```python
from build123d import *

# Parameters (mm, degrees)
BOSS_EXTRUDE1_DEPTH = 10
FILLET1_R           = 2


with BuildPart() as part:
    # Sketch1 → Boss-Extrude1 (new body)
    with BuildSketch(Plane.XY):
        with BuildLine():
            ThreePointArc((-10.758537028, -9.344323465), (-14.25, 0), (-10.758537028, 9.344323465))
            Line((-10.758537028, 9.344323465), (-15, 13.585786438))
            Line((-15, 13.585786438), (-15, -13.585786438))
            Line((-15, -13.585786438), (-10.758537028, -9.344323465))
        make_face()
        with BuildLine():
            ThreePointArc((-9.344323465, -10.758537028), (-10.076271632, -10.076271632), (-10.758537028, -9.344323465))
            Line((-10.758537028, -9.344323465), (-15, -13.585786438))
            Line((-15, -13.585786438), (-15, -15))
            Line((-15, -15), (-13.585786438, -15))
            Line((-13.585786438, -15), (-9.344323465, -10.758537028))
        make_face()
        with BuildLine():
            ThreePointArc((9.344323465, -10.758537028), (0, -14.25), (-9.344323465, -10.758537028))
            Line((-9.344323465, -10.758537028), (-13.585786438, -15))
            Line((-13.585786438, -15), (13.585786438, -15))
            Line((13.585786438, -15), (9.344323465, -10.758537028))
        make_face()
        with BuildLine():
            Line((15, -15), (15, -13.585786438))
            Line((15, -13.585786438), (10.758537028, -9.344323465))
            ThreePointArc((10.758537028, -9.344323465), (10.076271632, -10.076271632), (9.344323465, -10.758537028))
            Line((9.344323465, -10.758537028), (13.585786438, -15))
            Line((13.585786438, -15), (15, -15))
        make_face()
        with BuildLine():
            Line((15, 13.585786438), (10.758537028, 9.344323465))
            ThreePointArc((10.758537028, 9.344323465), (13.348626383, 4.987652121), (14.25, 0))
            ThreePointArc((14.25, 0), (13.348626383, -4.987652121), (10.758537028, -9.344323465))
            Line((10.758537028, -9.344323465), (15, -13.585786438))
            Line((15, -13.585786438), (15, 13.585786438))
        make_face()
        with BuildLine():
            Line((15, 15), (13.585786438, 15))
            Line((13.585786438, 15), (9.344323465, 10.758537028))
            ThreePointArc((9.344323465, 10.758537028), (10.076271632, 10.076271632), (10.758537028, 9.344323465))
            Line((10.758537028, 9.344323465), (15, 13.585786438))
            Line((15, 13.585786438), (15, 15))
        make_face()
        with BuildLine():
            Line((13.585786438, 15), (-13.585786438, 15))
            Line((-13.585786438, 15), (-9.344323465, 10.758537028))
            ThreePointArc((-9.344323465, 10.758537028), (0, 14.25), (9.344323465, 10.758537028))
            Line((9.344323465, 10.758537028), (13.585786438, 15))
        make_face()
        with BuildLine():
            Line((-9.344323465, 10.758537028), (-13.585786438, 15))
            Line((-13.585786438, 15), (-15, 15))
            Line((-15, 15), (-15, 13.585786438))
            Line((-15, 13.585786438), (-10.758537028, 9.344323465))
            ThreePointArc((-10.758537028, 9.344323465), (-10.076271632, 10.076271632), (-9.344323465, 10.758537028))
        make_face()
        with BuildLine():
            Line((3.83436875, -5.248582312), (0, -1.414213562))
            Line((0, -1.414213562), (-3.83436875, -5.248582312))
            ThreePointArc((-3.83436875, -5.248582312), (0, -6.5), (3.83436875, -5.248582312))
        make_face()
        with BuildLine():
            Line((0, -1.414213562), (-1.414213562, 0))
            Line((-1.414213562, 0), (-5.248582312, -3.83436875))
            ThreePointArc((-5.248582312, -3.83436875), (-4.596194078, -4.596194078), (-3.83436875, -5.248582312))
            Line((-3.83436875, -5.248582312), (0, -1.414213562))
        make_face()
        with BuildLine():
            Line((-1.414213562, 0), (-5.248582312, 3.83436875))
            ThreePointArc((-5.248582312, 3.83436875), (-6.5, 0), (-5.248582312, -3.83436875))
            Line((-5.248582312, -3.83436875), (-1.414213562, 0))
        make_face()
        with BuildLine():
            Line((0, 1.414213562), (-3.83436875, 5.248582312))
            ThreePointArc((-3.83436875, 5.248582312), (-4.596194078, 4.596194078), (-5.248582312, 3.83436875))
            Line((-5.248582312, 3.83436875), (-1.414213562, 0))
            Line((-1.414213562, 0), (0, 1.414213562))
        make_face()
        with BuildLine():
            ThreePointArc((3.83436875, 5.248582312), (0, 6.5), (-3.83436875, 5.248582312))
            Line((-3.83436875, 5.248582312), (0, 1.414213562))
            Line((0, 1.414213562), (3.83436875, 5.248582312))
        make_face()
        with BuildLine():
            Line((3.83436875, 5.248582312), (0, 1.414213562))
            Line((0, 1.414213562), (1.414213562, 0))
            Line((1.414213562, 0), (5.248582312, 3.83436875))
            ThreePointArc((5.248582312, 3.83436875), (4.596194078, 4.596194078), (3.83436875, 5.248582312))
        make_face()
        with BuildLine():
            Line((5.248582312, 3.83436875), (1.414213562, 0))
            Line((1.414213562, 0), (5.248582312, -3.83436875))
            ThreePointArc((5.248582312, -3.83436875), (6.179230738, -2.01670709), (6.5, 0))
            ThreePointArc((6.5, 0), (6.179230738, 2.01670709), (5.248582312, 3.83436875))
        make_face()
        with BuildLine():
            Line((5.248582312, -3.83436875), (1.414213562, 0))
            Line((1.414213562, 0), (0, -1.414213562))
            Line((0, -1.414213562), (3.83436875, -5.248582312))
            ThreePointArc((3.83436875, -5.248582312), (4.596194078, -4.596194078), (5.248582312, -3.83436875))
        make_face()
        with BuildLine():
            Line((-3.83436875, 5.248582312), (-9.344323465, 10.758537028))
            ThreePointArc((-9.344323465, 10.758537028), (-10.076271632, 10.076271632), (-10.758537028, 9.344323465))
            Line((-10.758537028, 9.344323465), (-5.248582312, 3.83436875))
            ThreePointArc((-5.248582312, 3.83436875), (-4.596194078, 4.596194078), (-3.83436875, 5.248582312))
        make_face()
        with BuildLine():
            Line((10.758537028, -9.344323465), (5.248582312, -3.83436875))
            ThreePointArc((5.248582312, -3.83436875), (4.596194078, -4.596194078), (3.83436875, -5.248582312))
            Line((3.83436875, -5.248582312), (9.344323465, -10.758537028))
            ThreePointArc((9.344323465, -10.758537028), (10.076271632, -10.076271632), (10.758537028, -9.344323465))
        make_face()
        with BuildLine():
            ThreePointArc((10.758537028, 9.344323465), (10.076271632, 10.076271632), (9.344323465, 10.758537028))
            Line((9.344323465, 10.758537028), (3.83436875, 5.248582312))
            ThreePointArc((3.83436875, 5.248582312), (4.596194078, 4.596194078), (5.248582312, 3.83436875))
            Line((5.248582312, 3.83436875), (10.758537028, 9.344323465))
        make_face()
        with BuildLine():
            Line((-5.248582312, -3.83436875), (-10.758537028, -9.344323465))
            ThreePointArc((-10.758537028, -9.344323465), (-10.076271632, -10.076271632), (-9.344323465, -10.758537028))
            Line((-9.344323465, -10.758537028), (-3.83436875, -5.248582312))
            ThreePointArc((-3.83436875, -5.248582312), (-4.596194078, -4.596194078), (-5.248582312, -3.83436875))
        make_face()
        Polygon((1.414213562, 0), (0, 1.414213562), (-1.414213562, 0), (0, -1.414213562), align=None)
    extrude(amount=BOSS_EXTRUDE1_DEPTH)

    # Fillet1
    fillet1_edges = [part.edges().sort_by_distance(p)[0] for p in [
        (15, -15, 5),
        (-15, -15, 5),
        (-15, 15, 5),
        (15, 15, 5),
    ]]
    fillet(fillet1_edges, radius=FILLET1_R)


solid = part.part
```
Source: CAD feature listing. Evaluate the final solid. Frame: model axes, mm. A direction names the side the tool comes from. Round coordinates to 2 decimals unless told otherwise and drop trailing zeros. Loops run counter-clockwise (first coordinate to the right, second up) from the corner with the lowest first, then second, coordinate; pieces in that order, holes last. Notation, with made-up numbers: M 74,50 L 89,50 A21 ccw 89,74 Z; hole C 45.25,12 d8. An arc over 180 degrees is marked long. Use a Markdown table: item, result. Add a question column.
1. Section query C-C on x = -1. Return the cut outline in (y, z), then the cut area to 3 significant figures.
2. Line query: line 1 (Y direction, x = 0, z = 1.75); line 2 (X direction, y = 5.5, z = 0.5); line 3 (Y direction, x = -8.75, z = 2.5). Output: solid intervals per line, ascending.
3. Section query B-B on y = -10. Return the cut outline in (x, z).
4. Mould query, pull axis Y, two halves, no side actions, for faces 3 (the flat face through (0, 15, 5)), 4 (the cylindrical face through (-6.5, 0.1, 4.9)), 5 (the cylindrical face through (-14.4, -14.43, 5.07)). Classes: pulls with the +Y half, pulls with the -Y half, needs draft (parallel to the pull), parting line crosses it, or undercut.
5. Section query D-D on x = 7.5. Return the cut outline in (y, z), then the cut area to 3 significant figures.
6. Reachability of faces 1 (the cylindrical face through (-0.1, -6.5, 4.9)), 2 (the flat face through (0, -15, 5)) from +Z, -Z, +X, -X, +Y, -Y: full face, straight path, thin tool, end or side. Return the list, or none.
7. Section query A-A on z = 6.5. Return the cut outline in (x, y).
Reported:
| question | item | result |
|---|---|---|
| 1 | outline | M -15,0 L -14.21,0 L -14.21,10 L -15,10 Z; M -6.42,0 L 6.42,0 L 6.42,10 L -6.42,10 Z; M 14.21,0 L 15,0 L 15,10 L 14.21,10 Z |
| 1 | area | 144 mm² |
| 2 | line 1 | y = -15 to -14.25, -6.5 to 6.5, 14.25 to 15 |
| 2 | line 2 | x = -15 to -13.15, -6.91 to -4.09, -3.46 to 3.46, 4.09 to 6.91, 13.15 to 15 |
| 2 | line 3 | y = -15 to -11.25, -10.16 to -7.34, 7.34 to 10.16, 11.25 to 15 |
| 3 | outline | M -15,0 L -8.59,0 L -8.59,10 L -15,10 Z; M 8.59,0 L 15,0 L 15,10 L 8.59,10 Z |
| 4 | face 3 | pulls with the +Y half |
| 4 | face 4 | undercut |
| 4 | face 5 | pulls with the -Y half |
| 5 | outline | M -15,0 L -12.12,0 L -12.12,10 L -15,10 Z; M -8.91,0 L -6.09,0 L -6.09,10 L -8.91,10 Z; M 6.09,0 L 8.91,0 L 8.91,10 L 6.09,10 Z; M 12.12,0 L 15,0 L 15,10 L 12.12,10 Z |
| 5 | area | 114 mm² |
| 6 | face 1 | +Z, -Z |
| 6 | face 2 | +Z, -Z, +X, -X, -Y |
| 7 | outline | M -15,-13 A2 ccw -13,-15 L 13,-15 A2 ccw 15,-13 L 15,13 A2 ccw 13,15 L -13,15 A2 ccw -15,13 Z; hole M -10.76,-9.34 L -5.25,-3.83 A6.5 cw -5.25,3.83 L -10.76,9.34 A14.25 ccw Z; hole M -9.34,-10.76 A14.25 ccw 9.34,-10.76 L 3.83,-5.25 A6.5 cw -3.83,-5.25 Z; hole M -9.34,10.76 L -3.83,5.25 A6.5 cw 3.83,5.25 L 9.34,10.76 A14.25 ccw Z; hole M 5.25,-3.83 L 10.76,-9.34 A14.25 ccw 10.76,9.34 L 5.25,3.83 A6.5 cw Z |
